Input: dimensioned drawing with shaded views. Units: mm. Origin: part minimum x, y, z. A direction names the side the tool comes from. Coordinates: 2 decimals unless noted, no trailing zeros. Loops run counter-clockwise (first coordinate to the right, second up) from the corner with the lowest first, then second, coordinate; pieces in that order, holes last.
(1) Line query: L1, parallel to Y at x = 3, z = 1.45; L2, parallel to Y at x = 10, z = 31; L3, parallel to X at y = 21.5, z = 18.5. Output: solid intervals per line, ascending.
(2) Section B-B, the plane y = 10. Return loops of the section in (x, z).
(3) Section C-C, the plane x = 2.25. Return loops of the section in (y, z).
(4) Set-up query: the marked faces 1 and 2. Return all of +Z, -Z, +X, -X, +Y, -Y with unobstructed straight access to the full face (end or side cutting, diameter ignored); none if empty.
(5) Section A-A, the plane z = 41. Return loops of the section in (x, y), then the cut area to 3 significant figures.
(6) Contact query for flat-ended pins moving along their axis: P1, Ø2.5, axis at y = 6.5, z = 22.5, coming from the +X side; P2, Ø1.5, axis at x = 2.5, y = 28, coming from the -Z side; P3, Ø17.5, axis at y = 20, z = 17.5, coming from the +X side; P4, Ø2.5, axis at x = 3, y = 10.5, coming from the -Z side. Output: stop coordinate, or through.
(7) Section D-D, the plane y = 19.5. Return loops of the section in (x, z), then the cut area to 3 significant figures.
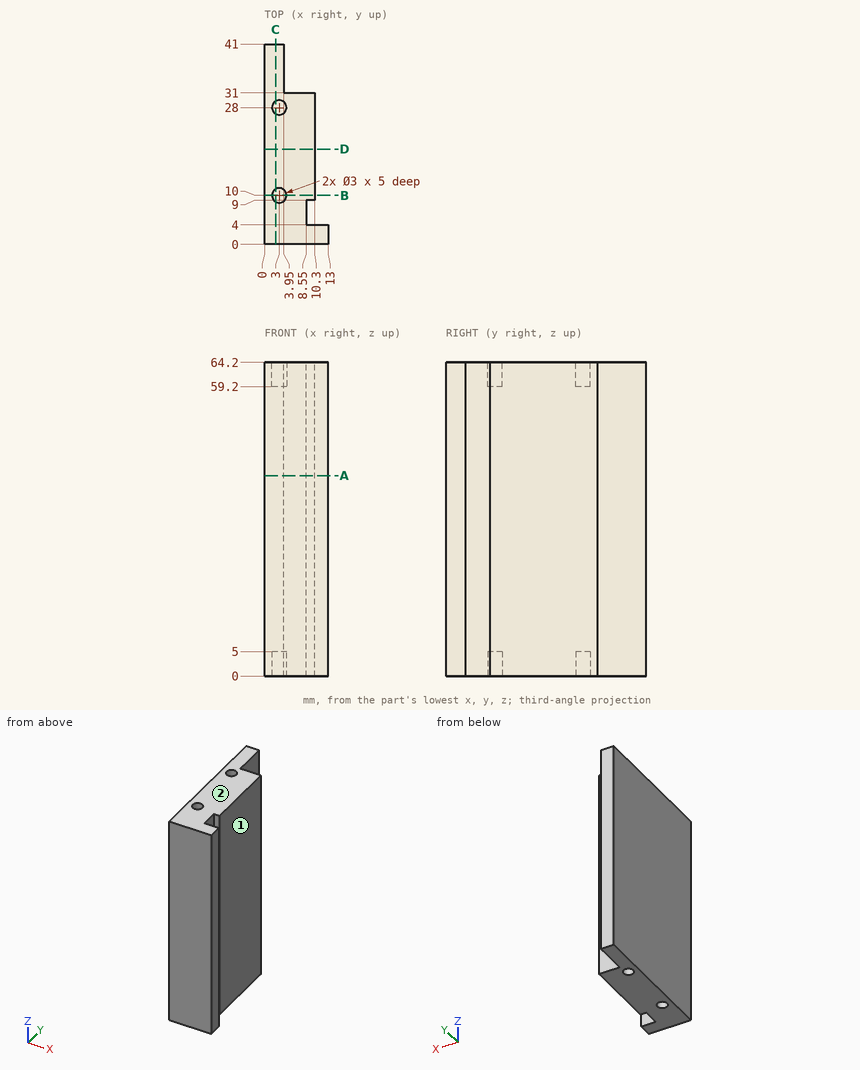
Report:
1. L1: y = 0 to 8.5, 11.5 to 26.5, 29.5 to 41
1. L2: y = 0 to 4, 9 to 31
1. L3: x = 0 to 10.3
2. outline: (0, 0) - (1.5, 0) - (1.5, 5) - (4.5, 5) - (4.5, 0) - (10.3, 0) - (10.3, 64.2) - (4.5, 64.2) - (4.5, 59.2) - (1.5, 59.2) - (1.5, 64.2) - (0, 64.2) - close
3. outline: (0, 0) - (8.7, 0) - (8.7, 5) - (11.3, 5) - (11.3, 0) - (26.7, 0) - (26.7, 5) - (29.3, 5) - (29.3, 0) - (41, 0) - (41, 64.2) - (29.3, 64.2) - (29.3, 59.2) - (26.7, 59.2) - (26.7, 64.2) - (11.3, 64.2) - (11.3, 59.2) - (8.7, 59.2) - (8.7, 64.2) - (0, 64.2) - close
4. face 1: +Z, -Z, +X, +Y
4. face 2: +Z, +X, -X, +Y, -Y
5. outline: (0, 0) - (13, 0) - (13, 4) - (8.55, 4) - (8.55, 9) - (10.3, 9) - (10.3, 31) - (3.95, 31) - (3.95, 41) - (0, 41) - close
5. area: 361 mm2
6. P1: stops at x = 8.55
6. P2: stops at z = 5
6. P3: stops at x = 10.3
6. P4: stops at z = 0
7. outline: (0, 0) - (10.3, 0) - (10.3, 64.2) - (0, 64.2) - close
7. area: 661 mm2
